Check sheet for the drawn part. Datum: minimum x, y, z corner. Units: mm. Give positions to 0.01 mm unless a question says otherwise; leave off trailing zeros. Order: outer loops, then holes, each group sorted by start corner. A loop starts at its lowest first (then second) coordinate and runs counter-clockwise, first axis right, second up.
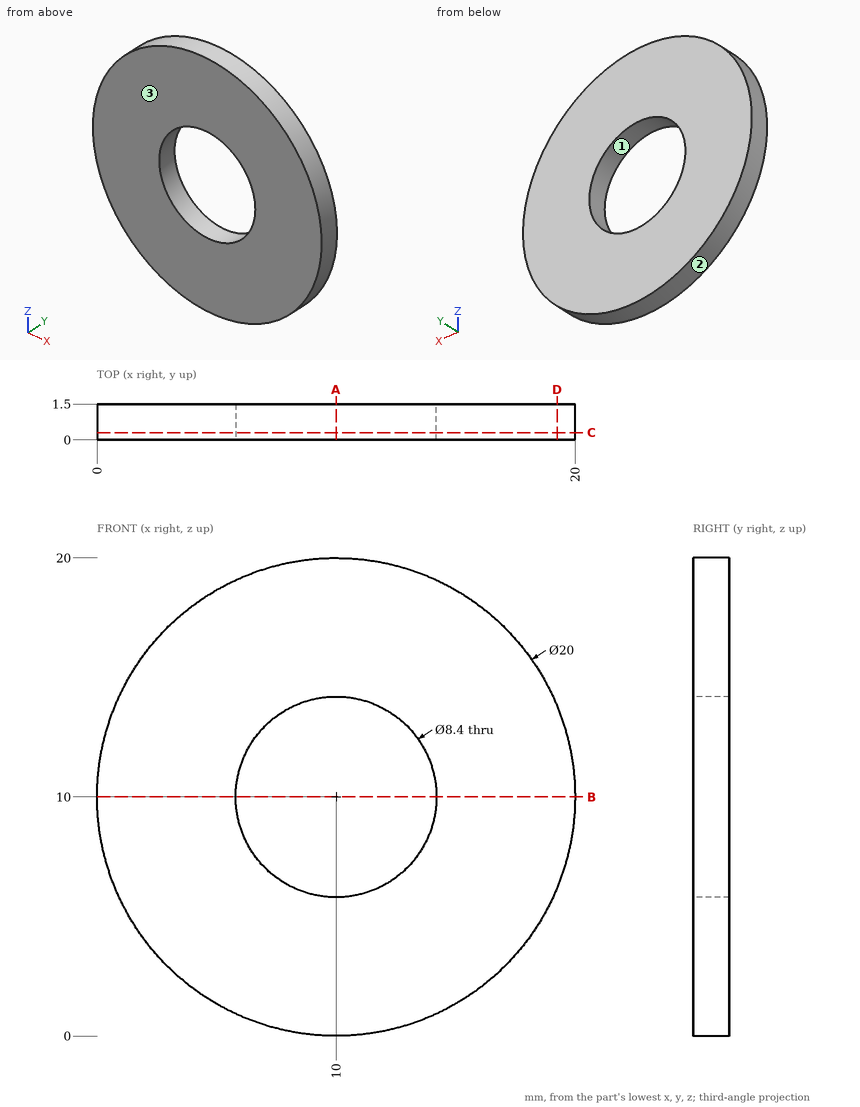
Item 1: Sectioned sample at B-B (z = 10). Enter the section's corners in (x, y), and give its area (3 significant figures).
Reported:
outline: (0, 0) - (5.8, 0) - (5.8, 1.5) - (0, 1.5) - close; (14.2, 0) - (20, 0) - (20, 1.5) - (14.2, 1.5) - close
area: 17.4 mm2
Item 2: Sectioned sample at A-A (x = 10). Enter the section's corners in (y, z), and give its area (3 significant figures).
Reported:
outline: (0, 0) - (1.5, 0) - (1.5, 5.8) - (0, 5.8) - close; (0, 14.2) - (1.5, 14.2) - (1.5, 20) - (0, 20) - close
area: 17.4 mm2
Item 3: Sectioned sample at C-C (y = 0.3). Enter the section's corners in (x, z).
Reported:
outline: circle Ø20 at (10, 10); hole circle Ø8.4 at (10, 10)
Item 4: Scan lines: L1, parallel to X at y = 1.15, z = 10; L2, parallel to X at y = 1.45, z = 13.5. Record each from-to range of solid material in increasing order.
Reported:
L1: x = 0 to 5.8, 14.2 to 20
L2: x = 0.63 to 7.68, 12.32 to 19.37
Item 5: Gauge pin test, flat end, axial feed: pin 1 (5 mm diameter, centred on x = 10, z = 10, fed in from +Y). Record the tip position at first contact, or that the pin passes through.
Reported:
pin 1: passes through
Item 6: Draft check along Z on the marked faces 1, 2 and 3. Enter one of: released by +Z, released by -Z, zero draft, split by the parting line, or undercut.
Reported:
face 1: undercut
face 2: split by the parting line
face 3: zero draft
Item 7: Sectioned sample at D-D (x = 19.25). Enter the section's corners in (y, z).
Reported:
outline: (0, 6.2) - (1.5, 6.2) - (1.5, 13.8) - (0, 13.8) - close
